from build123d import *

# Parameters (mm, degrees)
F0_W           = 6.35
F0_H           = 19.685
F0_R           = 2.38125
F1_DEPTH       = 3.048
F3_ANGLE_START = 10
F3_ANGLE       = 349
F4_W           = 6.35
F4_H           = 19.685
F4_R           = 2.38125
F5_DEPTH       = 6.35


with BuildPart() as f1:
    # F0 (on Right) → F1 (new body)
    with BuildSketch(Plane.YZ):
        with Locations((-3.175, 9.8425)):
            Rectangle(F0_W, F0_H)
        with Locations((-3.175, 16.51)):
            Circle(F0_R, mode=Mode.SUBTRACT)
    extrude(amount=F1_DEPTH)

    # F2 (on face) → F3 (revolve)
    with BuildSketch(Plane.YZ.offset(3.048), mode=Mode.PRIVATE) as f3_sk:
        with BuildLine():
            ThreePointArc((-0.79375, 6.35), (-4.8587980227, 8.0337980227), (-3.175, 3.96875))
            ThreePointArc((-3.175, 3.96875), (-1.4912019773, 4.6662019773), (-0.79375, 6.35))
        make_face()
    revolve(f3_sk.sketch.rotate(Axis((3.048, -5.2748635836, -6.35), (0, -1, 0)), F3_ANGLE_START), axis=Axis((3.048, -5.2748635836, -6.35), (0, -1, 0)), revolution_arc=F3_ANGLE)

    # F4 (on face) → F5 (join)
    with BuildSketch(Plane.YZ.offset(3.048)):
        with Locations((-3.175, 9.8425)):
            Rectangle(F4_W, F4_H)
        with Locations((-3.175, 16.51)):
            Circle(F4_R, mode=Mode.SUBTRACT)
    extrude(amount=F5_DEPTH)


solid = f1.part
CAD build for the part. Positions are in the model's coordinates, mm. A direction names the side the tool comes from. Give positions to 0.01 mm unless a question says otherwise; leave off trailing zeros. Write each loop counter-clockwise with the first axis right and the second up, starting at its lowest first coordinate (ties: lowest second). Pieces come first, ordered by that corner, then holes. Notation, with made-up numbers: (25, 6.25) - (60, 6.25) arc R7 ccw to (60, 16.25) - close; hole circle Ø10 at (51, 22). An arc over 180 degrees is marked (long way). Put each result on its own line as item: value.
(1) Saw through at B-B (y = -4). List the corners of the cut face in (x, z) (3 decimals), then the cut area to 3 significant figures.
Working result:
outline: (0, 8.269) arc R14.934 ccw (long way) to (9.398, 7.166) - (9.398, 14.276) - (0, 14.276) - close; (0, 18.744) - (9.398, 18.744) - (9.398, 19.685) - (0, 19.685) - close; hole (0, 0) - (0, 3.663) arc R10.466 ccw (long way) to (9.398, 1.97) - (9.398, 0) - close
area: 456 mm^2
(2) Tool access for faces 3 (the flat face through (5, -3, 0)), 4 (the flat face through (5, -3, 19.685)): list every direction of +Z, -Z, +X, -X, +Y, -Y with a clear straight run to the whole face (end or side of a thin tool).
Working result:
face 3: +Y, -Y
face 4: +Z, +X, -X, +Y, -Y
(3) Saw through at C-C (z = 1). Count the separate pieces of the cut face and the enclosed holes in it, then the cut area to 3 significant figures.
Working result:
separate pieces: 3
enclosed holes: 0
area: 104 mm^2
(4) Saw through at A-A (z = 16.51). List the corners of the cut face in (x, y), then the cut area to 3 significant figures.
Working result:
outline: (0, -6.35) - (9.4, -6.35) - (9.4, -5.56) - (0, -5.56) - close; (0, -0.79) - (9.4, -0.79) - (9.4, 0) - (0, 0) - close
area: 14.9 mm^2
(5) Drop flat-ended pins along their axis: pin 1 Ø10 at (x, z) = (-4.5, -15.5) entering from +Y; pin 2 Ø8 at (x, z) = (4, -12.5) entering from -Y; pin 3 Ø3 at (x, y) = (8.5, -4) entering from -Z; pin 4 Ø3 at (y, z) = (-4, 10) entering from +X. Give the stop position or say it passes through.
Working result:
pin 1: y = -0.79
pin 2: through
pin 3: z = -20.86
pin 4: x = 9.4
(6) Pull direction X, two halves, no side cores. Call faces 1 (the flat face through (5, -6.35, 10)), 2 (the flat face through (0, -3, 10)): released by +X, released by -X, zero draft, split by the parting line, or undercut.
Working result:
face 1: zero draft
face 2: undercut
(7) Wall check: L1, parallel to Z at x = 4, y = -2 (3 decimals); L2, parallel to Z at x = 3.5, y = -1.75 (3 decimals); L3, parallel to X at y = -0.5, z = 12. Give the ranges that are in metal, low to high.
Working result:
L1: -21.09 to -16.936, 0 to 14.439, 18.581 to 19.685
L2: -20.951 to -17.133, 0 to 14.602, 18.418 to 19.685
L3: 0 to 9.4
